The listing builds one solid part. Answer for the finished solid, in the listing's coordinates (mm). A direction names the side the tool comes from. Give positions to 0.01 mm unless a question says otherwise; leave off trailing zeros. Write each loop counter-clockwise with the first axis right and the second up, starting at its lowest first coordinate (ties: lowest second). Pieces come first, ordered by that corner, then holes. Notation, with made-up numbers: M 86,-25 L 139,-25 A20 cw 139,-6 Z; hole C -34.5,-26.75 d4. An arc over 180 degrees is marked long. Return JSON: item names as keys, results as strings.
from build123d import *

# Parameters (mm, degrees)
SKETCH8_W                       = 35
SKETCH8_H                       = 30
BOSS_EXTRUDE7_DEPTH             = 80
SKETCH10_R                      = 15
CUT_EXTRUDE3_DEPTH              = 18.5
CUT_EXTRUDE3_DEPTH_BACK         = 18.5
SKETCH11_W                      = 38.336381606
SKETCH11_H                      = 16.50007926
CUT_EXTRUDE4_DEPTH              = 18.5
CUT_EXTRUDE4_DEPTH_BACK         = 18.5
SKETCH12_W                      = 33.824881692
SKETCH12_H                      = 7.5
CUT_EXTRUDE5_DEPTH              = 18.5
CUT_EXTRUDE5_DEPTH_BACK         = 18.5
SKETCH13_W                      = 45.541829225
SKETCH13_H                      = 41.48776408
CUT_EXTRUDE6_DEPTH              = 18.5
CUT_EXTRUDE6_DEPTH_BACK         = 18.5
SKETCH15_W                      = 35
SKETCH15_H                      = 7.5
BOSS_EXTRUDE9_DEPTH             = 2
CUT_EXTRUDE7_DEPTH              = 2
SKETCH18_R                      = 3.2
CUT_EXTRUDE10_DEPTH             = 7.74996037
CUT_EXTRUDE10_DEPTH_BACK        = 6.4
CUT_EXTRUDE11_REACH             = 8.75
SKETCH19_R                      = 3.4
CUT_EXTRUDE11_DIRECTION_2_DEPTH = 4.9


with BuildPart() as part:
    # Sketch8 → Boss-Extrude7 (new body)
    with BuildSketch(Plane(origin=(0, 0, 0), x_dir=(1, 0, 0), z_dir=(0, 1, 0))):
        Rectangle(SKETCH8_W, SKETCH8_H)
    extrude(amount=BOSS_EXTRUDE7_DEPTH)

    # Sketch10 → Cut-Extrude3 (cut, two sides)
    with BuildSketch(Plane(origin=(0, 0, 0), x_dir=(0, 0, -1), z_dir=(1, 0, 0))) as cut_extrude3_sk:
        with Locations((0, 40)):
            Circle(SKETCH10_R)
    extrude(amount=CUT_EXTRUDE3_DEPTH, mode=Mode.SUBTRACT)
    extrude(cut_extrude3_sk.sketch, amount=-CUT_EXTRUDE3_DEPTH_BACK, mode=Mode.SUBTRACT)

    # Sketch11 → Cut-Extrude4 (cut, two sides)
    with BuildSketch(Plane(origin=(0, 0, 0), x_dir=(0, 0, -1), z_dir=(1, 0, 0))) as cut_extrude4_sk:
        with Locations((0, 40)):
            Rectangle(SKETCH11_W, SKETCH11_H)
    extrude(amount=CUT_EXTRUDE4_DEPTH, mode=Mode.SUBTRACT)
    extrude(cut_extrude4_sk.sketch, amount=-CUT_EXTRUDE4_DEPTH_BACK, mode=Mode.SUBTRACT)

    # Sketch12 → Cut-Extrude5 (cut, two sides)
    with BuildSketch(Plane(origin=(0, 0, 0), x_dir=(0, 0, -1), z_dir=(1, 0, 0))) as cut_extrude5_sk:
        with Locations((0.439040256, 3.75)):
            Rectangle(SKETCH12_W, SKETCH12_H)
    extrude(amount=CUT_EXTRUDE5_DEPTH, mode=Mode.SUBTRACT)
    extrude(cut_extrude5_sk.sketch, amount=-CUT_EXTRUDE5_DEPTH_BACK, mode=Mode.SUBTRACT)

    # Sketch13 → Cut-Extrude6 (cut, two sides)
    with BuildSketch(Plane(origin=(0, 0, 0), x_dir=(0, 0, -1), z_dir=(1, 0, 0))) as cut_extrude6_sk:
        with Locations((-6.569234617, 60.808180877)):
            Rectangle(SKETCH13_W, SKETCH13_H)
    extrude(amount=CUT_EXTRUDE6_DEPTH, mode=Mode.SUBTRACT)
    extrude(cut_extrude6_sk.sketch, amount=-CUT_EXTRUDE6_DEPTH_BACK, mode=Mode.SUBTRACT)

    # Sketch15 → Boss-Extrude9 (add)
    with BuildSketch(Plane(origin=(0, 7.5, 0), x_dir=(-1, 0, 0), z_dir=(0, -1, 0))):
        with Locations((0, -18.75)):
            Rectangle(SKETCH15_W, SKETCH15_H)
        with Locations((0, 18.75)):
            Rectangle(SKETCH15_W, SKETCH15_H)
    extrude(amount=-BOSS_EXTRUDE9_DEPTH)

    # Sketch16 → Cut-Extrude7 (cut)
    with BuildSketch(Plane(origin=(0, 7.5, 0), x_dir=(-1, 0, 0), z_dir=(0, -1, 0))):
        with BuildLine():
            Line((10, -20.863517543), (-10, -20.863517543))
            ThreePointArc((-10, -20.863517543), (-12, -18.863517543), (-10, -16.863517543))
            Line((-10, -16.863517543), (10, -16.863517543))
            ThreePointArc((10, -16.863517543), (12, -18.863517543), (10, -20.863517543))
        make_face()
        with BuildLine():
            Line((10, 16.803450623), (-10, 16.803450623))
            ThreePointArc((-10, 16.803450623), (-12, 18.803450623), (-10, 20.803450623))
            Line((-10, 20.803450623), (10, 20.803450623))
            ThreePointArc((10, 20.803450623), (12, 18.803450623), (10, 16.803450623))
        make_face()
    extrude(amount=-CUT_EXTRUDE7_DEPTH, mode=Mode.SUBTRACT)

    # Sketch18 → Cut-Extrude10 (cut, two sides)
    with BuildSketch(Plane(origin=(0, 25, 0), x_dir=(1, 0, 0), z_dir=(0, 1, 0))) as cut_extrude10_sk:
        Circle(SKETCH18_R)
        with Locations((10, 0)):
            Circle(SKETCH18_R)
        with Locations((-10, 0)):
            Circle(SKETCH18_R)
    extrude(amount=CUT_EXTRUDE10_DEPTH, mode=Mode.SUBTRACT)
    extrude(cut_extrude10_sk.sketch, amount=-CUT_EXTRUDE10_DEPTH_BACK, mode=Mode.SUBTRACT)

    # Sketch19 → Cut-Extrude11 (cut, up to next)
    with BuildSketch(Plane(origin=(0, 25, 0), x_dir=(1, 0, 0), z_dir=(0, 1, 0)), mode=Mode.PRIVATE) as cut_extrude11_sk1:
        with Locations((-10, -10)):
            Circle(SKETCH19_R)
    cut_extrude11_tool1 = extrude(cut_extrude11_sk1.sketch, amount=CUT_EXTRUDE11_REACH, mode=Mode.PRIVATE) & part.part
    add(cut_extrude11_tool1.solids().sort_by_distance((-10, 25, 10))[0], mode=Mode.SUBTRACT)
    # Sketch19 → Cut-Extrude11 (cut, up to next)
    with BuildSketch(Plane(origin=(0, 25, 0), x_dir=(1, 0, 0), z_dir=(0, 1, 0)), mode=Mode.PRIVATE) as cut_extrude11_sk2:
        with Locations((0, -10)):
            Circle(SKETCH19_R)
    cut_extrude11_tool2 = extrude(cut_extrude11_sk2.sketch, amount=CUT_EXTRUDE11_REACH, mode=Mode.PRIVATE) & part.part
    add(cut_extrude11_tool2.solids().sort_by_distance((0, 25, 10))[0], mode=Mode.SUBTRACT)
    # Sketch19 → Cut-Extrude11 (cut, up to next)
    with BuildSketch(Plane(origin=(0, 25, 0), x_dir=(1, 0, 0), z_dir=(0, 1, 0)), mode=Mode.PRIVATE) as cut_extrude11_sk3:
        with Locations((10, -10)):
            Circle(SKETCH19_R)
    cut_extrude11_tool3 = extrude(cut_extrude11_sk3.sketch, amount=CUT_EXTRUDE11_REACH, mode=Mode.PRIVATE) & part.part
    add(cut_extrude11_tool3.solids().sort_by_distance((10, 25, 10))[0], mode=Mode.SUBTRACT)
    # Sketch19 → Cut-Extrude11 (cut, up to next)
    with BuildSketch(Plane(origin=(0, 25, 0), x_dir=(1, 0, 0), z_dir=(0, 1, 0)), mode=Mode.PRIVATE) as cut_extrude11_sk4:
        with Locations((-10, 10)):
            Circle(SKETCH19_R)
    cut_extrude11_tool4 = extrude(cut_extrude11_sk4.sketch, amount=CUT_EXTRUDE11_REACH, mode=Mode.PRIVATE) & part.part
    add(cut_extrude11_tool4.solids().sort_by_distance((-10, 25, -10))[0], mode=Mode.SUBTRACT)
    # Sketch19 → Cut-Extrude11 (cut, up to next)
    with BuildSketch(Plane(origin=(0, 25, 0), x_dir=(1, 0, 0), z_dir=(0, 1, 0)), mode=Mode.PRIVATE) as cut_extrude11_sk5:
        with Locations((0, 10)):
            Circle(SKETCH19_R)
    cut_extrude11_tool5 = extrude(cut_extrude11_sk5.sketch, amount=CUT_EXTRUDE11_REACH, mode=Mode.PRIVATE) & part.part
    add(cut_extrude11_tool5.solids().sort_by_distance((0, 25, -10))[0], mode=Mode.SUBTRACT)
    # Sketch19 → Cut-Extrude11 (cut, up to next)
    with BuildSketch(Plane(origin=(0, 25, 0), x_dir=(1, 0, 0), z_dir=(0, 1, 0)), mode=Mode.PRIVATE) as cut_extrude11_sk6:
        with Locations((10, 10)):
            Circle(SKETCH19_R)
    cut_extrude11_tool6 = extrude(cut_extrude11_sk6.sketch, amount=CUT_EXTRUDE11_REACH, mode=Mode.PRIVATE) & part.part
    add(cut_extrude11_tool6.solids().sort_by_distance((10, 25, -10))[0], mode=Mode.SUBTRACT)

    # Sketch19 → Cut-Extrude11 direction 2 (cut)
    with BuildSketch(Plane(origin=(0, 25, 0), x_dir=(1, 0, 0), z_dir=(0, 1, 0))):
        with Locations((-10, -10)):
            Circle(SKETCH19_R)
        with Locations((0, -10)):
            Circle(SKETCH19_R)
        with Locations((10, -10)):
            Circle(SKETCH19_R)
        with Locations((-10, 10)):
            Circle(SKETCH19_R)
        with Locations((0, 10)):
            Circle(SKETCH19_R)
        with Locations((10, 10)):
            Circle(SKETCH19_R)
    extrude(amount=-CUT_EXTRUDE11_DIRECTION_2_DEPTH, mode=Mode.SUBTRACT)


solid = part.part
Item 1: A cutting plane is placed at D-D, the plane z = -10. Write down the section's boundary in (x, y).
Geometry results:
{"outline": "M -17.5,7.5 L 17.5,7.5 L 17.5,28.82 L 13.4,28.82 L 13.4,20.1 L 6.6,20.1 L 6.6,28.82 L 3.4,28.82 L 3.4,20.1 L -3.4,20.1 L -3.4,28.82 L -6.6,28.82 L -6.6,20.1 L -13.4,20.1 L -13.4,28.82 L -17.5,28.82 Z"}
Item 2: A cutting plane is placed at B-B, the plane z = 18. Write down the section's boundary in (x, y).
Geometry results:
{"outline": "M -17.5,7.5 L -11.8,7.5 L -11.8,9.5 L -17.5,9.5 Z; M 11.8,7.5 L 17.5,7.5 L 17.5,9.5 L 11.8,9.5 Z"}
Item 3: A cutting plane is placed at A-A, the plane x = -15. Write down the section's boundary in (y, z), plus the area to 3 significant figures.
Geometry results:
{"outline": "M 7.5,-22.5 L 9.5,-22.5 L 9.5,-15 L 31.75,-15 L 31.75,-12.53 A15 cw 31.75,12.53 L 31.75,15 L 9.5,15 L 9.5,22.5 L 7.5,22.5 Z", "area": "638 mm2"}
Item 4: Determine the mould class of faces 4 (the flat face through (-17.5, 17, 0)), 5 (the flat face through (0, 20.1, -10)), 6 (the flat face through (0, 7.5, 0)) for opening direction X: +X half, -X half, draft (parallel to the pull), parting line (faces both ways), or undercut.
Geometry results:
{"face 4": "-X half", "face 5": "undercut", "face 6": "draft"}
Item 5: Given pin 1 Ø2 at (x, z) = (-9, -9) entering from +Y; pin 2 Ø5 at (x, y) = (9, 17) entering from +Z; pin 3 Ø8 at (x, z) = (6.5, -20) entering from +Y, each flat-ended and moving along its own axis, determine where each tip first touches the part or whether it passes through.
Geometry results:
{"pin 1": "stops at y = 20.1", "pin 2": "stops at z = 15", "pin 3": "stops at y = 9.5"}
Item 6: Find the intervals of material crossed by line 1 (Z direction, x = 0, y = 23.25); line 2 (X direction, y = 23, z = 10); line 3 (X direction, y = 23, z = 0), in increasing order.
Geometry results:
{"line 1": "z = -15 to -13.4, -6.6 to -3.2, 3.2 to 6.6, 13.4 to 15", "line 2": "x = -17.5 to -13.4, -6.6 to -3.4, 3.4 to 6.6, 13.4 to 17.5", "line 3": "x = -17.5 to -13.2, -6.8 to -3.2, 3.2 to 6.8, 13.2 to 17.5"}
Item 7: A cutting plane is placed at C-C, the plane y = 24. Count the separate pieces of the cut face and the enclosed holes in it, plus the area to 3 significant figures.
Geometry results:
{"separate pieces": "1", "enclosed holes": "9", "area": "736 mm2"}
Item 8: Which of the six approach directions +Z, -Z, +X, -X, +Y, -Y give full straight-line access (tool end or side, diameter ignored) to faces 1 (the flat face through (0, 20, 15)), 2 (the flat face through (0, 8, 20.864)), 3 (the cylindrical face through (-0.44, 24.55, -13.37))?
Geometry results:
{"face 1": "+Z, +X, -X, +Y", "face 2": "+Y, -Y", "face 3": "+Y"}
